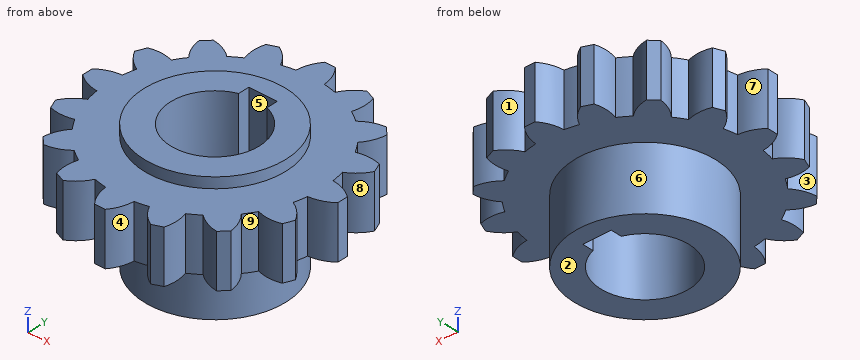
from build123d import *

# Parameters (mm, degrees)
SKETCH1_R           = 30
BOSS_EXTRUDE1_DEPTH = 15
SKETCH2_R           = 20
BOSS_EXTRUDE2_DEPTH = 3
BOSS_EXTRUDE3_START = 18
SKETCH3_R           = 20
BOSS_EXTRUDE3_DEPTH = 18
CUT_EXTRUDE1_DEPTH  = 56.641710973
BOSS_EXTRUDE5_DEPTH = 7.5


with BuildPart() as part:
    # Sketch1 → Boss-Extrude1 (new body)
    with BuildSketch(Plane.XY):
        Circle(SKETCH1_R)
    extrude(amount=BOSS_EXTRUDE1_DEPTH)

    # Sketch2 → Boss-Extrude2 (add)
    with BuildSketch(Plane.XY.offset(15)):
        Circle(SKETCH2_R)
    extrude(amount=BOSS_EXTRUDE2_DEPTH)

    # Sketch3 → Boss-Extrude3 (add)
    with BuildSketch(Plane(origin=(0, 0, 0), x_dir=(-1, 0, 0), z_dir=(0, 0, -1)).offset(BOSS_EXTRUDE3_START)):
        with Locations(Location((0, 0, 0), (0, 0, 180))):
            Circle(SKETCH3_R)
    extrude(amount=-BOSS_EXTRUDE3_DEPTH)

    # Sketch4 → Cut-Extrude1 (cut, through all)
    with BuildSketch(Plane(origin=(0, 0, -18), x_dir=(-1, 0, 0), z_dir=(0, 0, -1))):
        with BuildLine():
            Line((-4, 15), (4, 15))
            Line((4, 15), (4, 11.842719282))
            ThreePointArc((4, 11.842719282), (0, -12.5), (-4, 11.842719282))
            Line((-4, 11.842719282), (-4, 15))
        make_face()
    extrude(amount=-CUT_EXTRUDE1_DEPTH, mode=Mode.SUBTRACT)

    # Sketch5 → Boss-Extrude5 (add, symmetric)
    with BuildSketch(Plane.XY.offset(7.5)):
        with BuildLine():
            Line((-1.5, 36), (1.5, 36))
            ThreePointArc((1.5, 36), (3.242504384, 33.062509074), (4, 29.732137495))
            ThreePointArc((4, 29.732137495), (0, 30), (-4, 29.732137495))
            ThreePointArc((-4, 29.732137495), (-3.242504384, 33.062509074), (-1.5, 36))
        make_face()
        with BuildLine():
            Line((12.390784266, 33.833688319), (15.162422864, 32.685638022))
            ThreePointArc((15.162422864, 32.685638022), (15.64815789, 29.30492272), (15.073514558, 25.93817956))
            ThreePointArc((15.073514558, 25.93817956), (11.480502971, 27.716385975), (7.682478298, 28.999647019))
            ThreePointArc((7.682478298, 28.999647019), (9.656791021, 31.786628134), (12.390784266, 33.833688319))
        make_face()
        with BuildLine():
            Line((24.395183951, 26.516504294), (26.516504295, 24.395183951))
            ThreePointArc((26.516504295, 24.395183951), (25.671521208, 21.085927531), (23.852223166, 18.195368917))
            ThreePointArc((23.852223166, 18.195368917), (21.213203436, 21.213203436), (18.195368917, 23.852223166))
            ThreePointArc((18.195368917, 23.852223166), (21.085927531, 25.671521208), (24.395183951, 26.516504294))
        make_face()
        with BuildLine():
            Line((32.685638022, 15.162422864), (33.833688319, 12.390784266))
            ThreePointArc((33.833688319, 12.390784266), (31.786628135, 9.656791021), (28.999647019, 7.682478298))
            ThreePointArc((28.999647019, 7.682478298), (27.716385975, 11.480502971), (25.93817956, 15.073514558))
            ThreePointArc((25.93817956, 15.073514558), (29.30492272, 15.64815789), (32.685638022, 15.162422864))
        make_face()
        with BuildLine():
            Line((36, 1.5), (36, -1.5))
            ThreePointArc((36, -1.5), (33.062509074, -3.242504384), (29.732137495, -4))
            ThreePointArc((29.732137495, -4), (30, 0), (29.732137495, 4))
            ThreePointArc((29.732137495, 4), (33.062509074, 3.242504384), (36, 1.5))
        make_face()
        with BuildLine():
            Line((33.833688319, -12.390784266), (32.685638022, -15.162422864))
            ThreePointArc((32.685638022, -15.162422864), (29.30492272, -15.64815789), (25.93817956, -15.073514558))
            ThreePointArc((25.93817956, -15.073514558), (27.716385975, -11.480502971), (28.999647019, -7.682478298))
            ThreePointArc((28.999647019, -7.682478298), (31.786628135, -9.656791021), (33.833688319, -12.390784266))
        make_face()
        with BuildLine():
            Line((26.516504295, -24.395183951), (24.395183951, -26.516504295))
            ThreePointArc((24.395183951, -26.516504295), (21.085927531, -25.671521208), (18.195368917, -23.852223166))
            ThreePointArc((18.195368917, -23.852223166), (21.213203436, -21.213203436), (23.852223166, -18.195368917))
            ThreePointArc((23.852223166, -18.195368917), (25.671521208, -21.085927531), (26.516504295, -24.395183951))
        make_face()
        with BuildLine():
            Line((15.162422864, -32.685638022), (12.390784266, -33.833688319))
            ThreePointArc((12.390784266, -33.833688319), (9.656791021, -31.786628135), (7.682478298, -28.999647019))
            ThreePointArc((7.682478298, -28.999647019), (11.480502971, -27.716385975), (15.073514558, -25.93817956))
            ThreePointArc((15.073514558, -25.93817956), (15.64815789, -29.30492272), (15.162422864, -32.685638022))
        make_face()
        with BuildLine():
            Line((1.5, -36), (-1.5, -36))
            ThreePointArc((-1.5, -36), (-3.242504384, -33.062509074), (-4, -29.732137495))
            ThreePointArc((-4, -29.732137495), (0, -30), (4, -29.732137495))
            ThreePointArc((4, -29.732137495), (3.242504384, -33.062509074), (1.5, -36))
        make_face()
        with BuildLine():
            Line((-12.390784266, -33.833688319), (-15.162422864, -32.685638022))
            ThreePointArc((-15.162422864, -32.685638022), (-15.64815789, -29.30492272), (-15.073514558, -25.93817956))
            ThreePointArc((-15.073514558, -25.93817956), (-11.480502971, -27.716385975), (-7.682478298, -28.999647019))
            ThreePointArc((-7.682478298, -28.999647019), (-9.656791021, -31.786628135), (-12.390784266, -33.833688319))
        make_face()
        with BuildLine():
            Line((-24.395183951, -26.516504295), (-26.516504295, -24.395183951))
            ThreePointArc((-26.516504295, -24.395183951), (-25.671521208, -21.085927531), (-23.852223166, -18.195368917))
            ThreePointArc((-23.852223166, -18.195368917), (-21.213203436, -21.213203436), (-18.195368917, -23.852223166))
            ThreePointArc((-18.195368917, -23.852223166), (-21.085927531, -25.671521208), (-24.395183951, -26.516504295))
        make_face()
        with BuildLine():
            Line((-32.685638022, -15.162422864), (-33.833688319, -12.390784266))
            ThreePointArc((-33.833688319, -12.390784266), (-31.786628135, -9.656791021), (-28.999647019, -7.682478298))
            ThreePointArc((-28.999647019, -7.682478298), (-27.716385975, -11.480502971), (-25.93817956, -15.073514558))
            ThreePointArc((-25.93817956, -15.073514558), (-29.30492272, -15.64815789), (-32.685638022, -15.162422864))
        make_face()
        with BuildLine():
            Line((-36, -1.5), (-36, 1.5))
            ThreePointArc((-36, 1.5), (-33.062509074, 3.242504384), (-29.732137495, 4))
            ThreePointArc((-29.732137495, 4), (-30, 0), (-29.732137495, -4))
            ThreePointArc((-29.732137495, -4), (-33.062509074, -3.242504384), (-36, -1.5))
        make_face()
        with BuildLine():
            Line((-33.833688319, 12.390784266), (-32.685638022, 15.162422864))
            ThreePointArc((-32.685638022, 15.162422864), (-29.30492272, 15.64815789), (-25.93817956, 15.073514558))
            ThreePointArc((-25.93817956, 15.073514558), (-27.716385975, 11.480502971), (-28.999647019, 7.682478298))
            ThreePointArc((-28.999647019, 7.682478298), (-31.786628135, 9.656791021), (-33.833688319, 12.390784266))
        make_face()
        with BuildLine():
            Line((-26.516504295, 24.395183951), (-24.395183951, 26.516504294))
            ThreePointArc((-24.395183951, 26.516504294), (-21.085927531, 25.671521208), (-18.195368917, 23.852223166))
            ThreePointArc((-18.195368917, 23.852223166), (-21.213203436, 21.213203436), (-23.852223166, 18.195368917))
            ThreePointArc((-23.852223166, 18.195368917), (-25.671521208, 21.085927531), (-26.516504295, 24.395183951))
        make_face()
        with BuildLine():
            Line((-15.162422864, 32.685638022), (-12.390784266, 33.833688319))
            ThreePointArc((-12.390784266, 33.833688319), (-9.656791021, 31.786628134), (-7.682478298, 28.999647019))
            ThreePointArc((-7.682478298, 28.999647019), (-11.480502971, 27.716385975), (-15.073514558, 25.93817956))
            ThreePointArc((-15.073514558, 25.93817956), (-15.64815789, 29.30492272), (-15.162422864, 32.685638022))
        make_face()
    extrude(amount=BOSS_EXTRUDE5_DEPTH, both=True)


solid = part.part
Check sheet for the modelled part. Datum: model origin and axes. Units: mm. Face numbers are marked on the shaded views. A direction names the side the tool comes from. Round coordinates to 2 decimals unless told otherwise and drop trailing zeros. Order: outer loops, then holes, each group sorted by start corner. A loop starts at its lowest first (then second) coordinate and runs counter-clockwise, first axis right, second up. Notation, with made-up numbers: M 51.5,44.25 L 64.5,44.25 A26 cw 64.5,78.25 Z; hole C 67.25,85 d11. An arc over 180 degrees is marked long. One line per item, written item: value. Start each with the question number.
1. Section check A-A on y = 0. Enter the section's corners in (x, z), and give its area (3 significant figures).
2. Section check B-B on x = 0. Enter the section's corners in (y, z).
3. Section check C-C on y = -31.5. Enter the section's corners in (x, z), and give its area (3 significant figures).
4. Section check D-D on z = -14. Enter the section's corners in (x, y), and give its area (3 significant figures).
5. Scan lines: line 1 along Y through (x, z) = (0, -5.5); line 2 along Y through (x, z) = (0, 3.5); line 3 along Z through (x, y) = (17, -23). Record each from-to range of solid material in increasing order.
6. Access from +Z, -Z, +X, -X, +Y, -Y to the whole of each face (thin tool, end or side, straight path). Record for the marked faces 1, 2, 3, 4 and 5.
7. Release check for a two-part mould opening along X. For the marked faces 6, 7, 8 and 9 record: released by +X, released by -X, zero draft, split by the parting line, or undercut.
8. Gauge pin test, flat ends, axial feed: P1, Ø1.6, axis at y = 14, z = 5.5, coming from the -X side; P2, Ø2, axis at x = -8.5, z = -3, coming from the -Y side; P3, Ø12, axis at x = 23, z = 10.5, coming from the -Y side. Record the tip position at first contact, or that the pin passes through.
Results found:
1. outline: M -36,0 L -20,0 L -20,-18 L -12.5,-18 L -12.5,18 L -20,18 L -20,15 L -36,15 Z; M 12.5,-18 L 20,-18 L 20,0 L 36,0 L 36,15 L 20,15 L 20,18 L 12.5,18 Z
1. area: 1,020 mm^2
2. outline: M -36,0 L -20,0 L -20,-18 L -12.5,-18 L -12.5,18 L -20,18 L -20,15 L -36,15 Z; M 15,-18 L 20,-18 L 20,0 L 36,0 L 36,15 L 20,15 L 20,18 L 15,18 Z
3. outline: M -15.46,0 L -9.39,0 L -9.39,15 L -15.46,15 Z; M -3.73,0 L 3.73,0 L 3.73,15 L -3.73,15 Z; M 9.39,0 L 15.46,0 L 15.46,15 L 9.39,15 Z
3. area: 294 mm^2
4. outline: C 0,0 d40; hole M -4,11.84 A12.5 ccw long 4,11.84 L 4,15 L -4,15 Z
4. area: 744 mm^2
5. line 1: -20 to -12.5, 15 to 20
5. line 2: -36 to -12.5, 15 to 36
5. line 3: 0 to 15
6. face 1: +Z, -Z, +Y
6. face 2: -Z, +X, -X, +Y, -Y
6. face 3: +Z, -Z, -X
6. face 4: +Z, -Z, -Y
6. face 5: +Z, -Z
7. face 6: split by the parting line
7. face 7: released by -X
7. face 8: released by +X
7. face 9: undercut
8. P1: x = -33.5
8. P2: y = -18.54
8. P3: y = -26.52
